Here's how the part is built. I have some questions about the finished solid (model axes, mm). Face numbers are marked on the shaded views. A direction names the side the tool comes from. Round coordinates to 2 decimals unless told otherwise and drop trailing zeros. Loops run counter-clockwise (first coordinate to the right, second up) from the corner with the lowest first, then second, coordinate; pieces in that order, holes last. Notation, with made-up numbers: (4.5, -11.75) -> (22.5, -11.75) arc R20 ccw to (22.5, -3.75) -> close; hole circle Ø7 at (-29, -32). An arc over 180 degrees is marked (long way). One line per item, written item: value. Start each with the question number.
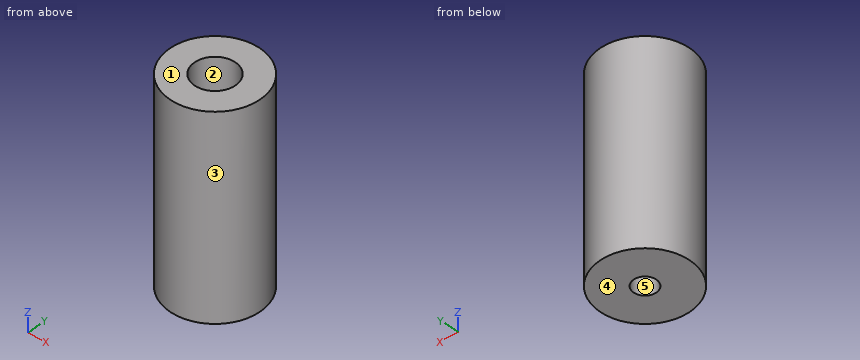
Solid Edge part; units mm, degrees
sketch "Sketch1" plane through (0, 0, 0) normal (0, 0, 1) x (1, 0, 0)
  circle A0 centre (0, 0) radius 2.15
extrude "Protrusion1" add sketch "Sketch1" along normal blind 3
sketch "Sketch2" plane through (0, 0, 0) normal (0, 0, 1) x (1, 0, 0)
  circle A0 centre (0, 0) radius 4.75
  circle A1 centre (0, 0) radius 2.15
extrude "ExtrudedProtrusion_2" add sketch "Sketch2" along normal blind 15
sketch "Sketch3" plane through (0, 0, 0) normal (0, 0, 1) x (1, 0, 0)
  circle A0 centre (0, 0) radius 4.75
  circle A1 centre (0, 0) radius 1.2
extrude "ExtrudedProtrusion_3" add sketch "Sketch3" against normal blind 6
Q1. I want a section at C-C on z = -0.5. Please give me the cut outline in (x, y).
Q2. I want a section at A-A on y = 0. Please give me the cut outline in (x, z).
Q3. If I drill on line 1 along Y through (x, z) = (0, 7.5); line 2 along Y through (x, z) = (0, -1.9); line 3 along X through (y, z) = (-0.25, 5), over which ranges is the centre line in solid material (lowest first)?
Q4. I want a section at D-D on z = 2.5. Please give me the cut outline in (x, y), plus the area to 3 significant figures.
Q5. Which directions (+Z, -Z, +X, -X, +Y, -Y) give clear straight access to the entire face, cutting with the end or side of a thin tool? Please do the marked faces 4 and 5.
Q6. If we mould it in two halves opening along X, with no side actions, what happens to the marked faces 1, 2 and 3? For each: released by +X, released by -X, zero draft, split by the parting line, or undercut.
Q7. Will these pins go through, and if not, where does the flat tip stop? P1, Ø1.9, axis at x = 0.5, y = 0, coming from the -Z side; P2, Ø4, axis at x = 2.5, z = -1.5, coming from the +Y side; P3, Ø1.4, axis at x = 0, y = 0, coming from the +Z side; P4, Ø4, axis at y = -2.5, z = 6.5, coming from the +X side.
Answers below:
1. outline: circle Ø9.5 at (0, 0); hole circle Ø2.4 at (0, 0)
2. outline: (-4.75, -6) -> (-1.2, -6) -> (-1.2, 0) -> (1.2, 0) -> (1.2, -6) -> (4.75, -6) -> (4.75, 15) -> (2.15, 15) -> (2.15, 3) -> (-2.15, 3) -> (-2.15, 15) -> (-4.75, 15) -> close
3. line 1: y = -4.75 to -2.15, 2.15 to 4.75
3. line 2: y = -4.75 to -1.2, 1.2 to 4.75
3. line 3: x = -4.74 to -2.14, 2.14 to 4.74
4. outline: circle Ø9.5 at (0, 0)
4. area: 70.9 mm^2
5. face 4: -Z, +X, -X, +Y, -Y
5. face 5: -Z
6. face 1: zero draft
6. face 2: undercut
6. face 3: split by the parting line
7. P1: stops at z = -6
7. P2: stops at y = 4.72
7. P3: stops at z = 3
7. P4: stops at x = 4.72
